from build123d import *

# Parameters (mm, degrees)
F0_R     = 8
F1_DEPTH = 3.5


# Not quite as in the source:
# - the program builds the solid bodies; features that only make, move or delete a surface that nothing else refers to are left out


with BuildPart() as f1:
    # F0 (on Top) → F1 (new body)
    with BuildSketch(Plane.XY):
        with BuildLine():
            ThreePointArc((0, -12.5), (-12.5, 0), (0, 12.5))
            Line((0, 12.5), (-35, 12.5))
            Line((-35, 12.5), (-116.3887844346, 2.5067138408))
            Line((-116.3887844346, 2.5067138408), (-116.3887844346, -2.5067138408))
            Line((-116.3887844346, -2.5067138408), (-35, -12.5))
            Line((-35, -12.5), (0, -12.5))
        make_face()
        with BuildLine():
            ThreePointArc((0, -12.5), (8.8388347648, -8.8388347648), (12.5, 0))
            ThreePointArc((12.5, 0), (8.8388347648, 8.8388347648), (0, 12.5))
            ThreePointArc((0, 12.5), (-12.5, 0), (0, -12.5))
        make_face()
        Circle(F0_R, mode=Mode.SUBTRACT)
    extrude(amount=F1_DEPTH)


solid = f1.part
The model under review builds one solid part; all positions refer to its coordinate system, in mm. Give positions to 0.01 mm unless a question says otherwise; leave off trailing zeros. Loops run counter-clockwise (first coordinate to the right, second up) from the corner with the lowest first, then second, coordinate; pieces in that order, holes last. Notation, with made-up numbers: (75, 65.5) -> (108, 65.5) arc R21 cw to (108, 96.5) -> close; hole circle Ø1 at (59, 40.5). An arc over 180 degrees is marked (long way). Put each result on its own line as item: value. Start each with the question number.
1. We need section A-A on z = 1.85. State the section outline as (x, y) points, then the cut area to 3 significant figures.
2. We need section B-B on x = -82. State the section outline as (y, z) points.
3. Mouldability with a two-part tool opening along X and no side actions: class faces 1 (the face through (-116.389, 0, 2)), 2 (the face through (-1.73, -7.81, 1.73)), 3 (the face through (-17, 12.5, 2)) as released by +X, released by -X, zero draft, split by the parting line, or undercut.
4. Wall thickness on probe 1 along Y at (x, z) = (0, 1.45); probe 2 along Y at (x, z) = (5, 0.45) (3 decimals); probe 3 along X at (y, z) = (1.5, 1.6): over which ranges is each line inside the solid? List them lowest first.
5. Clearance check with a flat-ended pin moving along its axis: P1, Ø2, axis at x = -43.5, y = 2.5, coming from the -Z side. State where the tip first meets the part, or that it passes through.
6. We need section C-C on y = 10. State the section outline as (x, z) points.
Determined:
1. outline: (-116.39, -2.51) -> (-35, -12.5) -> (0, -12.5) arc R12.5 ccw to (0, 12.5) -> (-35, 12.5) -> (-116.39, 2.51) -> close; hole circle Ø16 at (0, 0)
1. area: 2,140 mm^2
2. outline: (-6.73, 0) -> (6.73, 0) -> (6.73, 3.5) -> (-6.73, 3.5) -> close
3. face 1: released by -X
3. face 2: undercut
3. face 3: zero draft
4. probe 1: -12.5 to -8, 8 to 12.5
4. probe 2: -11.456 to -6.245, 6.245 to 11.456
4. probe 3: -116.39 to -7.86, 7.86 to 12.41
5. P1: z = 0
6. outline: (-55.36, 0) -> (7.5, 0) -> (7.5, 3.5) -> (-55.36, 3.5) -> close
